Here's the drawing with two shaded views (mm, measured from the low corner). I have some questions. A direction names the side the tool comes from. Round coordinates to 2 decimals unless told otherwise and drop trailing zeros. Loops run counter-clockwise (first coordinate to the right, second up) from the corner with the lowest first, then second, coordinate; pieces in that order, holes last.
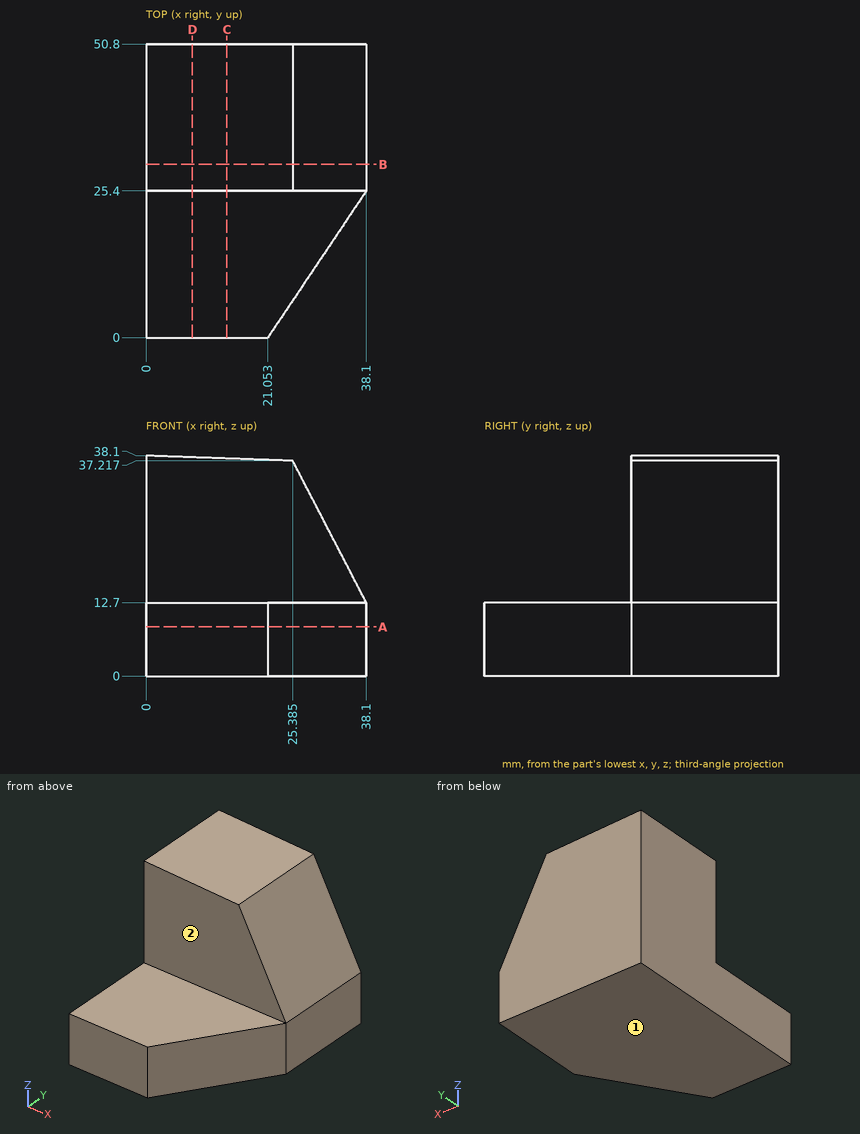
Item 1: If I drill on line 1 along Z through (x, y) = (18.5, 3); line 2 along Y through (x, z) = (20.5, 18); line 3 along Z through (x, y) = (13, 27), over which ranges is the centre line in solid material (lowest first)?
Results list:
line 1: z = 0 to 12.7
line 2: y = 25.4 to 50.8
line 3: z = 0 to 37.65
Item 2: If we section it at C-C, the plane x = 14: Please give me the cut outline in (y, z), then the cut area to 3 significant figures.
Results list:
outline: (0, 0) - (50.8, 0) - (50.8, 37.61) - (25.4, 37.61) - (25.4, 12.7) - (0, 12.7) - close
area: 1,280 mm2
Item 3: If we section it at B-B, the plane y = 30: Please give me the cut outline in (x, z) (1 decimal).
Results list:
outline: (0, 0) - (38.1, 0) - (38.1, 12.7) - (25.4, 37.2) - (0, 38.1) - close
Item 4: If we section it at D-D, the plane x = 8: Please give me the cut outline in (y, z).
Results list:
outline: (0, 0) - (50.8, 0) - (50.8, 37.82) - (25.4, 37.82) - (25.4, 12.7) - (0, 12.7) - close
Item 5: If we section it at A-A, the plane z = 8.5: Please give me the cut outline in (x, y).
Results list:
outline: (0, 0) - (21.05, 0) - (38.1, 25.4) - (38.1, 50.8) - (0, 50.8) - close
Item 6: Will these pins go through, and if not, where does the flat tip stop? pin 1 (5 mm diameter, centred on x = 20.5, z = 23.5, fed in from -Y); pin 2 (12 mm diameter, centred on y = 16.5, z = 34, fed in from +X); pin 3 (8 mm diameter, centred on y = 30, z = 30.5, fed in from +X); pin 4 (1 mm diameter, centred on x = 21.5, y = 10.5, fed in from +Z).
Results list:
pin 1: stops at y = 25.4
pin 2: passes through
pin 3: stops at x = 30.94
pin 4: stops at z = 12.7
Item 7: For the marked faces 1 and 2, which set-ups out of +Z, -Z, +X, -X, +Y, -Y let a thin tool reach every point of the face, with its end or its side?
Results list:
face 1: -Z, +X, -X, +Y, -Y
face 2: +Z, +X, -X, -Y
